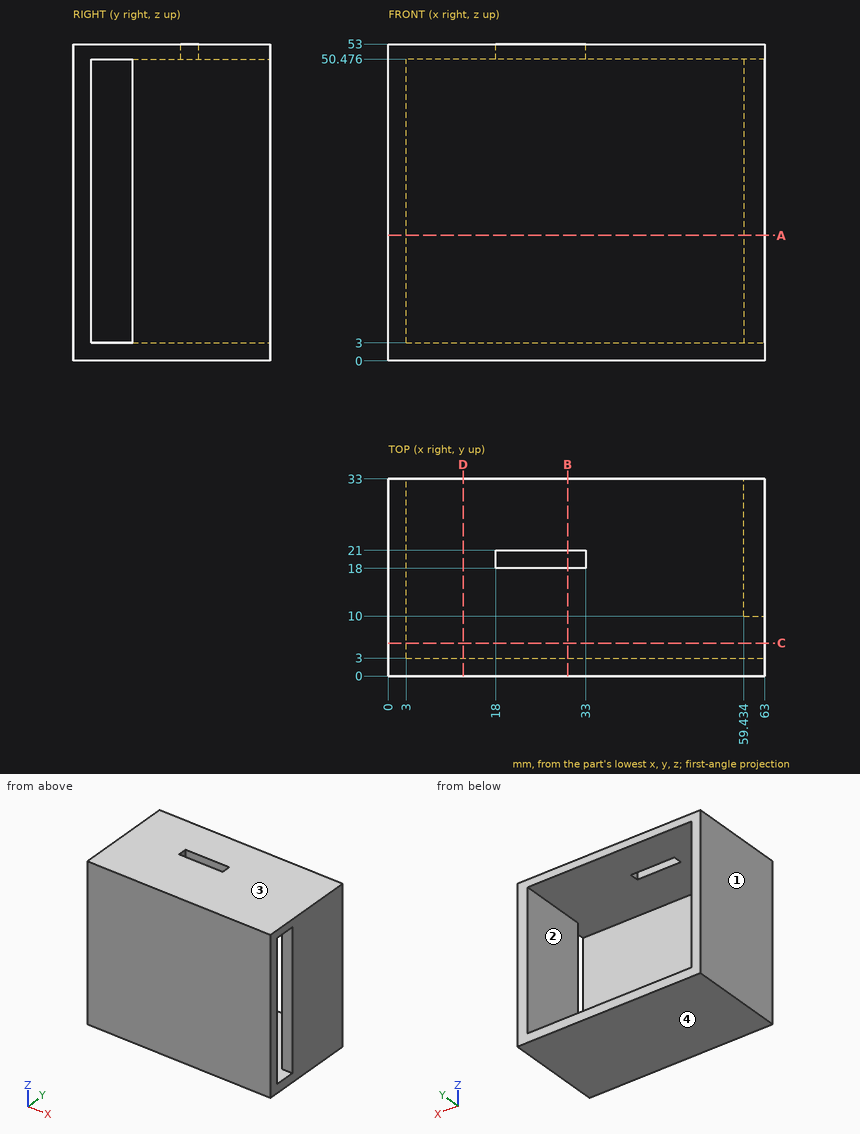
Could you check a few things on this drawing? It's one solid part, dimensions in mm from its lowest x, y, z. Give positions to 0.01 mm unless a question says otherwise; leave off trailing zeros. Loops run counter-clockwise (first coordinate to the right, second up) from the corner with the lowest first, then second, coordinate; pieces in that order, holes last. Notation, with made-up numbers: M 48.5,-2.75 L 76.5,-2.75 A28 ccw 76.5,26.25 Z; hole C -31.5,25 d8. An arc over 180 degrees is marked long. Return JSON: item names as keys, results as strings.
Item 1: I'm going to push flat-ended pins straight in: pin 1 Ø1 at (x, z) = (51, 40) entering from +Y; pin 2 Ø1 at (y, z) = (8.5, 17.5) entering from +X. Where does each tip first touch, or does it pass through?
A:
{"pin 1": "stops at y = 3", "pin 2": "stops at x = 3"}
Item 2: Imagine slicing it at C-C on y = 5.5. List the corners of the cut face in (x, z) for me.
A:
{"outline": "M 0,0 L 63,0 L 63,3 L 3,3 L 3,50.48 L 63,50.48 L 63,53 L 0,53 Z"}
Item 3: Imagine slicing it at A-A on z = 21. List the corners of the cut face in (x, y) for me.
A:
{"outline": "M 0,0 L 63,0 L 63,3 L 3,3 L 3,33 L 0,33 Z; M 59.43,10 L 63,10 L 63,33 L 59.43,33 Z"}
Item 4: Thinking about a two-plate mould opening in Z: for the marked faces 1, 2, 3 and 4, which applies, released by +Z, released by -Z, zero draft, split by the parting line, or undercut?
A:
{"face 1": "zero draft", "face 2": "undercut", "face 3": "released by +Z", "face 4": "released by -Z"}
Item 5: Please list where these lines run through material, in increasing order: line 1 (X direction, y = 17, z = 31.5); line 2 (Z direction, x = 41.5, y = 14); line 3 (Y direction, x = 60.5, z = 44).
A:
{"line 1": "x = 0 to 3, 59.43 to 63", "line 2": "z = 0 to 3, 50.48 to 53", "line 3": "y = 0 to 3, 10 to 33"}
Item 6: Imagine slicing it at B-B on x = 30. List the corners of the cut face in (y, z) for me.
A:
{"outline": "M 0,0 L 33,0 L 33,3 L 3,3 L 3,50.48 L 18,50.48 L 18,53 L 0,53 Z; M 21,50.48 L 33,50.48 L 33,53 L 21,53 Z"}
Item 7: Imagine slicing it at D-D on x = 12.5. List the corners of the cut face in (y, z) for me, then the cut area to 3 significant figures.
A:
{"outline": "M 0,0 L 33,0 L 33,3 L 3,3 L 3,50.48 L 33,50.48 L 33,53 L 0,53 Z", "area": "325 mm^2"}
